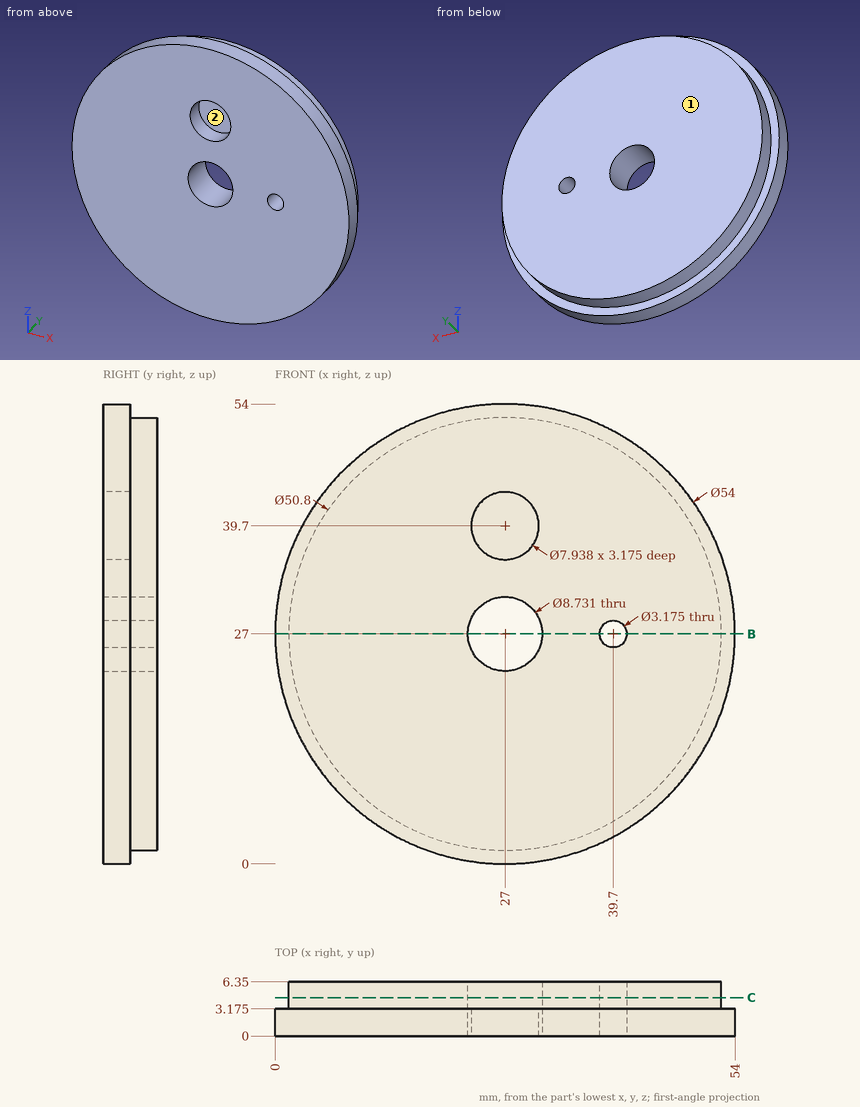
Input: dimensioned drawing with shaded views. Units: mm. Origin: part minimum x, y, z. Coordinates: 2 decimals unless noted, no trailing zeros. Write each loop counter-clockwise with the first axis right and the second up, starting at its lowest first coordinate (ties: lowest second). Pieces come first, ordered by that corner, then holes. Notation, with made-up numbers: (62, -24.75) -> (89, -24.75) arc R18 ccw to (89, -1.75) -> close; hole circle Ø1 at (-24, -3.5). An arc over 180 degrees is marked (long way). Return JSON: item names as keys, results as strings. Group by question number.
1) Contact query for flat-ended pins moving along their axis: P1, Ø3, axis at x = 46, y = 3.5, coming from the -Z side; P2, Ø4, axis at x = 27.5, z = 39, coming from the -Y side (1 decimal); P3, Ø4, axis at x = 16.5, z = 12, coming from the -Y side; P4, Ø1, axis at x = 28.5, y = 5.5, coming from the +Z side. Output: stop coordinate, or through.
2) Section query B-B, the plane z = 27. State how many separate pieces and enclosed holes the cut face has, plus the area to 3 significant figures.
3) Ray query, line 1 along X through (y, z) = (3, 27) (1 decimal); line 2 along Z through (x, y) = (27, 4.5) (1 decimal); line 3 along Z through (x, y) = (28.5, 1.75) (1 decimal). Return the intervals inside material, ascending.
4) Section query C-C, the plane y = 4.5. Return loops of the section in (x, z) (1 decimal), plus the area to 3 significant figures.
5) Mould query, pull axis Z, two halves, no side actions, for the marked faces 1 and 2. Classes: +Z half, -Z half, draft (parallel to the pull), parting line (faces both ways), or undercut.
From the geometry:
{
 "1": {"P1": "z = 6.47", "P2": "y = 3.2", "P3": "y = 0", "P4": "z = 52.38"},
 "2": {"separate pieces": "3", "enclosed holes": "0", "area": "257 mm²"},
 "3": {"line 1": "0 to 22.6, 31.4 to 38.1, 41.3 to 54", "line 2": "1.6 to 22.6, 31.4 to 52.4", "line 3": "0 to 22.9, 31.1 to 36, 43.4 to 54"},
 "4": {"outline": "circle Ø50.8 at (27, 27); hole circle Ø8.7 at (27, 27); hole circle Ø3.2 at (39.7, 27)", "area": "1,960 mm²"},
 "5": {"face 1": "draft", "face 2": "undercut"}
}
